```python
from build123d import *

# Parameters (mm, degrees)
SCHIZZO1_R                   = 4
ESTRUSIONE_ESTRUSIONE1_DEPTH = 5.5


with BuildPart() as part:
    # Schizzo1 → Estrusione-Estrusione1 (new body)
    with BuildSketch(Plane.XY):
        with BuildLine():
            Line((-27.25, 0), (27.25, 0))
            ThreePointArc((27.25, 0), (28.75, -1.5), (27.25, -3))
            Line((27.25, -3), (10.69143351, -8))
            ThreePointArc((10.69143351, -8), (2.524901098, -17.966332655), (-7.2357096, -9.555))
            ThreePointArc((-7.2357096, -9.555), (-8.241759605, -7.493469312), (-10.410277522, -6.745421563))
            Line((-10.410277522, -6.745421563), (-31.25, -8))
            Line((-31.25, -8), (-27.25, 0))
        make_face()
        with Locations((1.7471616, -9)):
            Circle(SCHIZZO1_R, mode=Mode.SUBTRACT)
    extrude(amount=ESTRUSIONE_ESTRUSIONE1_DEPTH)


solid = part.part
```
Model file for the job. Use its own axes, mm. A direction names the side the tool comes from. Give positions to 0.01 mm unless a question says otherwise; leave off trailing zeros. Write each loop counter-clockwise with the first axis right and the second up, starting at its lowest first coordinate (ties: lowest second). Pieces come first, ordered by that corner, then holes. Notation, with made-up numbers: (-3.5, -1.5) - (8.5, -1.5) arc R23 cw to (8.5, 21.5) - close; hole circle Ø7 at (77.25, -1.75). An arc over 180 degrees is marked (long way). One line per question, with ' | ' between items. Start each with the question number.
(1) Slice it at D-D on x = 10. Write the cut outline in (y, z).
(2) 3-axis set-ups, long thin cutter, end or side, ignore diameter. For faces 4 (the face through (-29.3, -4.1, 2.7)), 5 (the face through (-20.684, -7.364, 2.712)): which of +Z, -Z, +X, -X, +Y, -Y reach the whole face in a straight line?
(3) Two-plate mould, pull along Y, no slides. Class faces 1 (the face through (3.59, -12.55, 2.71)), 2 (the face through (28.75, -1.47, 2.71)), 3 (the face through (0, 0, 3)): +Y half, -Y half, draft (parallel to the pull), parting line (faces both ways), or undercut.
(4) Slice it at C-C on y = -1.5. Write the cut outline in (x, z).
(5) Slice it at A-A on z = 2.25. Write the cut outline in (x, y) (3 decimals), plus the area to 3 significant figures.
(6) Pin check, flat tips, straight feed: P1, Ø6.5, axis at x = 1.75, y = -9, coming from the -Z side; P2, Ø1.5, axis at x = 15, z = 1.5, coming from the -Y side; P3, Ø1.5, axis at y = -3, z = 4.5, coming from the +X side. Stop position of each tip, or through.
(7) Wall check: line 1 along Y through (x, z) = (-10, 5.1); line 2 along X through (y, z) = (-9.5, 1.3); line 3 along Y through (x, z) = (3, 4.1). Give the ranges that are in metal, low to high. Write a range as from..to.
(8) Slice it at B-B on y = -7.25. Write the cut outline in (x, z) (3 decimals), plus the area to 3 significant figures.
Results below:
1) outline: (-12.59, 0) - (0, 0) - (0, 5.5) - (-12.59, 5.5) - close
2) face 4: +Z, -Z, -X, +Y | face 5: +Z, -Z, -Y
3) face 1: undercut | face 2: parting line | face 3: +Y half
4) outline: (-28, 0) - (28.75, 0) - (28.75, 5.5) - (-28, 5.5) - close
5) outline: (-31.25, -8) - (-10.41, -6.745) arc R3 cw to (-7.236, -9.555) arc R9 ccw (long way) to (10.691, -8) - (27.25, -3) arc R1.5 ccw to (27.25, 0) - (-27.25, 0) - close; hole circle Ø8 at (1.747, -9) | area: 494 mm^2
6) P1: through | P2: y = -6.93 | P3: x = 28.55
7) line 1: -6.75..0 | line 2: -7.24..-2.22, 5.72..10.73 | line 3: -17.91..-12.8, -5.2..0
8) outline: (-30.875, 0) - (-18.792, 0) - (-18.792, 5.5) - (-30.875, 5.5) - close; (-8.557, 0) - (-1.85, 0) - (-1.85, 5.5) - (-8.557, 5.5) - close; (5.344, 0) - (13.175, 0) - (13.175, 5.5) - (5.344, 5.5) - close | area: 146 mm^2
